```python
from build123d import *

# Parameters (mm, degrees)
F1_DEPTH = 90.5968919396
F2_R     = 13.402691555
F3_R     = 3.5726570055
F4_DEPTH = 36.660566926


with BuildPart() as f1:
    # F0 (on Front) → F1 (new body)
    with BuildSketch(Plane.XZ):
        Polygon((36.8415974081, 38.5606420045), (10.5619765818, 38.5606420045), (10.5619765818, 0), (36.8415974081, 1.5603324458), align=None)
    extrude(amount=F1_DEPTH)

    # F2
    f2_edges = [f1.edges().sort_by_distance(p)[0] for p in [
        (36.841597, -45.298446, 38.560642),
    ]]
    fillet(f2_edges, radius=F2_R)

    # F3 (on face) → F4 (join)
    with BuildSketch(Plane.XZ.offset(90.5968919396)):
        with Locations((23.4389058531, 25.1579504495)):
            Circle(F3_R)
    extrude(amount=F4_DEPTH)


solid = f1.part
```
Design review of the part built by this model. Coordinates are the model's own, in mm. A direction names the side the tool comes from. Give positions to 0.01 mm unless a question says otherwise; leave off trailing zeros. Write each loop counter-clockwise with the first axis right and the second up, starting at its lowest first coordinate (ties: lowest second). Pieces come first, ordered by that corner, then holes.
(1) Tool access review of faces 1 (the face through (36.842, -45, 13)), 2 (the face through (19.87, -108.67, 25.32)): name each direction out of +Z, -Z, +X, -X, +Y, -Y from which nothing blocks a thin tool from reaching the whole face with its end or side.
Checked values:
face 1: +Z, -Z, +X, +Y, -Y
face 2: -Y
(2) Add section B-B (x = 25.25). Give the boundary of the cut face in (y, z), and give its area (3 significant figures).
Checked values:
outline: (-127.26, 22.08) - (-90.6, 22.08) - (-90.6, 0.87) - (0, 0.87) - (0, 38.44) - (-90.6, 38.44) - (-90.6, 28.24) - (-127.26, 28.24) - close
area: 3,630 mm2
(3) Add section A-A (y = -48). Give the boundary of the cut face in (x, z), and give its area (3 significant figures).
Checked values:
outline: (10.56, 0) - (36.84, 1.56) - (36.84, 25.16) arc R13.4 ccw to (23.44, 38.56) - (10.56, 38.56) - close
area: 954 mm2
(4) Add section C-C (z = 17). Give the boundary of the cut face in (x, y).
Checked values:
outline: (10.56, -90.6) - (36.84, -90.6) - (36.84, 0) - (10.56, 0) - close
(5) Add section D-D (y = -111). Give the boundary of the cut face in (x, z).
Checked values:
outline: circle Ø7.15 at (23.44, 25.16)
(6) Wall thickness on line 1 along Y through (x, z) = (28.25, 15); line 2 along X through (y, z) = (-42, 26); line 3 along Z through (x, y) = (18.25, -51.5): over which ranges is each line inside the solid? List them lowest first.
Checked values:
line 1: y = -90.6 to 0
line 2: x = 10.56 to 36.82
line 3: z = 0.46 to 38.56
